Source: CAD feature listing. Evaluate the final solid. Frame: model axes, mm. Face numbers are marked on the shaded views. Give positions to 0.01 mm unless a question says otherwise; leave off trailing zeros. Write each loop counter-clockwise with the first axis right and the second up, starting at its lowest first coordinate (ties: lowest second). Pieces come first, ordered by that corner, then holes.
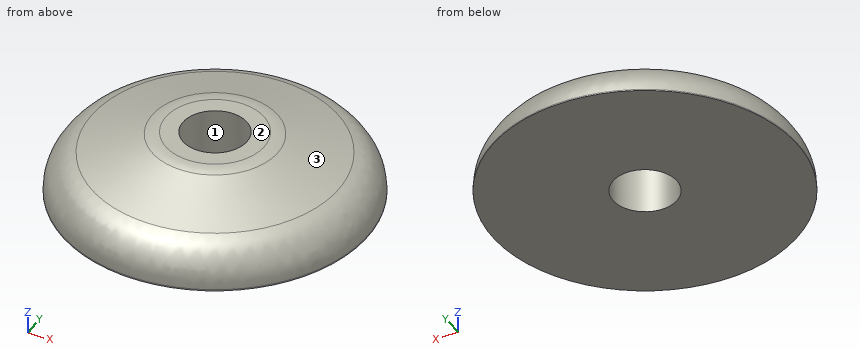
```python
from build123d import *

# Parameters (mm, degrees)
F0_R     = 14.25
F1_DEPTH = 6
F2_R     = 3
F3_DEPTH = 25
F4_SIZE2 = 3
F4_SIZE  = 9
F5_R     = 4


with BuildPart() as f1:
    # F0 (on Top) → F1 (new body)
    with BuildSketch(Plane.XY):
        Circle(F0_R)
    extrude(amount=F1_DEPTH)

    # F2 (on face) → F3 (cut)
    with BuildSketch(Plane.XY.offset(6)):
        Circle(F2_R)
    extrude(amount=-F3_DEPTH, mode=Mode.SUBTRACT)

    # F4
    f4_edges = [f1.edges().sort_by_distance(p)[0] for p in [
        (-14.25, 0, 6),
    ]]
    f4_side = f1.faces().sort_by_distance((-13.846949, 0, 6))[0]
    chamfer(f4_edges, length=F4_SIZE, length2=F4_SIZE2, reference=f4_side)

    # F5
    f5_edges = [f1.edges().sort_by_distance(p)[0] for p in [
        (-5.25, 0, 6),
        (-14.25, 0, 3),
    ]]
    fillet(f5_edges, radius=F5_R)


solid = f1.part
```
1. Contact query for flat-ended pins moving along their axis: P1, Ø2, axis at x = -1.5, y = -6, coming from the +Z side; P2, Ø10, axis at x = 5.5, y = -10, coming from the +Z side; P3, Ø8, axis at x = 10.5, y = -7.5, coming from the +Z side. Output: stop coordinate, or through.
2. Mould query, pull axis X, two halves, no side actions, for the marked faces 1, 2 and 3. Classes: +X half, -X half, draft (parallel to the pull), parting line (faces both ways), or undercut.
3. Cut plane A-A, the plane z = 5. Return the cut outline in (x, y).
4. Line query: L1, parallel to Y at x = -2.25, z = 0.75; L2, parallel to Y at x = 0, z = 2.15; L3, parallel to X at y = -4.75, z = 0.75. Output: solid intervals per line, ascending.
Response values:
1. P1: stops at z = 5.96
1. P2: stops at z = 5.61
1. P3: stops at z = 4.78
2. face 1: undercut
2. face 2: draft
2. face 3: parting line
3. outline: circle Ø16.5 at (0, 0); hole circle Ø6 at (0, 0)
4. L1: y = -14.02 to -1.98, 1.98 to 14.02
4. L2: y = -13.69 to -3, 3 to 13.69
4. L3: x = -13.38 to 13.38
